Work out the finished part from the listing and answer in its coordinate system (mm). Face numbers are marked on the shaded views. Give positions to 0.01 mm unless a question says otherwise; leave off trailing zeros. Loops run counter-clockwise (first coordinate to the right, second up) from the corner with the lowest first, then second, coordinate; pieces in that order, holes last. Notation, with made-up numbers: M -39,27.25 L 6,27.25 A24 ccw 6,65.25 Z; hole C 67.5,-22.75 d11. An arc over 180 degrees is marked long. Write item = value, one per line. Start each with the question number.
1. Flat-ended cylindrical pins translate along their axes: pin 1 Ø10 at (x, z) = (16, 155.5) entering from +Y; pin 2 Ø6 at (x, y) = (-18.5, -10) entering from -Z; pin 3 Ø7.5 at (x, y) = (-5.5, 2.5) entering from +Z. Find the tip coordinate at first contact, or state that the pin passes through.
2. Section C-C on y = -55.5 is taken. Determine the outline of the cut face in (x, z).
3. Consider L1, parallel to Y at x = 0, z = 9; L2, parallel to Y at x = 0, z = -1.25; L3, parallel to Y at x = 0, z = 11.2. Determine where each line is inside the solid, lowest interval first. Write a range as [from, to].
4. Section B-B on z = 20 is taken. Determine the outline of the cut face in (x, y), plus the area to 3 significant figures.
5. The mould has two halves that part along Y. Classify the marked faces 1 and 2: released by +Y, released by -Y, zero draft, split by the parting line, or undercut.
6. Section D-D on x = 22 is taken. Determine the outline of the cut face in (y, z).
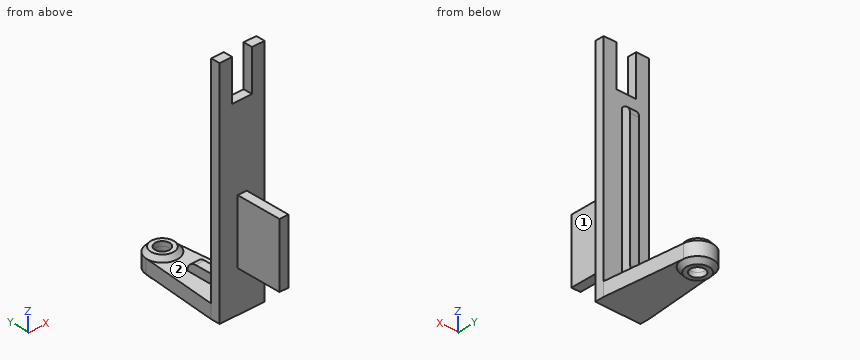
```python
from build123d import *

# Parameters (mm, degrees)
BOSS_EXTRUDE1_DEPTH = 7.5
SKETCH2_W           = 50
SKETCH2_H           = 10
BOSS_EXTRUDE2_DEPTH = 235
SKETCH4_W           = 70
SKETCH4_H           = 49.933850778
BOSS_EXTRUDE3_DEPTH = 5
SKETCH5_R           = 8
CUT_EXTRUDE1_DEPTH  = 21
SKETCH6_W           = 67.307350871
SKETCH6_H           = 68.73953257
CUT_EXTRUDE2_DEPTH  = 11


with BuildPart() as part:
    # Sketch1 → Boss-Extrude1 (new body, symmetric)
    with BuildSketch(Plane.XY):
        with BuildLine():
            Line((-25, -85), (-16.926566325, 1.57840186))
            ThreePointArc((-16.926566325, 1.57840186), (0, 17), (16.926566325, 1.57840186))
            Line((16.926566325, 1.57840186), (25, -85))
            Line((25, -85), (25, -95))
            Line((25, -95), (-25, -95))
            Line((-25, -95), (-25, -85))
        make_face()
    extrude(amount=BOSS_EXTRUDE1_DEPTH, both=True)

    # Sketch2 → Boss-Extrude2 (add)
    with BuildSketch(Plane.XY.offset(7.5)):
        with Locations((0, -90)):
            Rectangle(SKETCH2_W, SKETCH2_H)
    extrude(amount=BOSS_EXTRUDE2_DEPTH)

    # Sketch3 → Revolve1 (revolve)
    with BuildSketch(Plane(origin=(0, 0, 0), x_dir=(0, 0, -1), z_dir=(1, 0, 0)), mode=Mode.PRIVATE) as revolve1_sk:
        Polygon((-12.5, 8), (-12.5, 12.5), (-7.5, 17), (-7.5, 8), align=None)
        Polygon((12.5, 8), (7.5, 8), (7.5, 17), (12.5, 12.5), align=None)
    revolve(revolve1_sk.sketch.rotate(Axis((0, 0, 1025), (0, 0, -1)), 90), axis=Axis((0, 0, 1025), (0, 0, -1)))  # turned: the seam where the file's is

    # Sketch4 → Boss-Extrude3 (add, symmetric)
    with BuildSketch(Plane(origin=(0, 0, 0), x_dir=(0, 0, -1), z_dir=(1, 0, 0))):
        with BuildLine():
            Line((-17.509416808, -45), (-17.509416808, -65))
            ThreePointArc((-17.509416808, -65), (-20.438348996, -72.071067812), (-27.509416808, -75))
            Line((-27.509416808, -75), (-172.5, -75))
            ThreePointArc((-172.5, -75), (-179.571067812, -77.928932188), (-182.5, -85))
            Line((-182.5, -85), (-7.5, -85))
            Line((-7.5, -85), (-7.5, -35))
            Line((-7.5, -35), (-7.509416808, -35))
            ThreePointArc((-7.509416808, -35), (-14.58048462, -37.928932188), (-17.509416808, -45))
        make_face()
        with Locations((-72.5, -119.966925389)):
            Rectangle(SKETCH4_W, SKETCH4_H)
    extrude(amount=BOSS_EXTRUDE3_DEPTH, both=True)

    # Sketch5 → Cut-Extrude1 (cut, through all)
    with BuildSketch(Plane.XY.offset(7.5)):
        Circle(SKETCH5_R)
    extrude(amount=-CUT_EXTRUDE1_DEPTH, mode=Mode.SUBTRACT)

    # Sketch6 → Cut-Extrude2 (cut, symmetric)
    with BuildSketch(Plane(origin=(0, 0, 0), x_dir=(0, 0, -1), z_dir=(1, 0, 0))):
        with Locations((-231.153675436, -92.172536307)):
            Rectangle(SKETCH6_W, SKETCH6_H)
    extrude(amount=CUT_EXTRUDE2_DEPTH, both=True, mode=Mode.SUBTRACT)


solid = part.part
```
Verdict:
q1.pin_1 = -85
q1.pin_2 = -7.5
q1.pin_3 = 12.5
q2.outline = M -22.25,-7.5 L 22.25,-7.5 L 22.25,7.5 L 5,7.5 L 5,17.51 L -5,17.51 L -5,7.5 L -22.25,7.5 Z
q3.L1 = [-95, -35.11], [-15.65, -8], [8, 15.65]
q3.L2 = [-95, -8], [8, 17]
q3.L3 = [-95, -35.71], [-13.67, -8], [8, 13.67]
q4.outline = M -25,-95 L 25,-95 L 25,-85 L 5,-85 L 5,-71.6 L -5,-71.6 L -5,-85 L -25,-85 Z
q4.area = 634 mm2
q5.face_1 = zero draft
q5.face_2 = undercut
q6.outline = M -95,-7.5 L -52.83,-7.5 L -52.83,7.5 L -85,7.5 L -85,242.5 L -95,242.5 Z
